Check sheet for the modelled part. Datum: model origin and axes. Units: mm. A direction names the side the tool comes from. Coordinates: 2 decimals unless noted, no trailing zeros. Loops run counter-clockwise (first coordinate to the right, second up) from the corner with the lowest first, then second, coordinate; pieces in that order, holes last. Notation, with made-up numbers: M -10.75,4.5 L 40.25,4.5 A28 cw 40.25,31.5 Z; hole C -10,22.25 d2. An arc over 180 degrees is marked long. Return JSON: item names as keys, results as strings.
from build123d import *

# Parameters (mm, degrees)
CROQUIS1_W              = 60
CROQUIS1_H              = 25
SALIENTE_EXTRUIR1_DEPTH = 25
CROQUIS2_R              = 22
CORTAR_EXTRUIR1_DEPTH   = 25
CROQUIS3_W              = 39.331186887
CROQUIS3_H              = 32.545982132
CORTAR_EXTRUIR6_DEPTH   = 5
CROQUIS6_W              = 71.754194534
CROQUIS6_H              = 47.315533904
CORTAR_EXTRUIR7_DEPTH   = 5
CROQUIS7_W              = 50
CROQUIS7_H              = 25
SALIENTE_EXTRUIR2_DEPTH = 2
CORTAR_EXTRUIR9_DEPTH   = 38
CORTAR_EXTRUIR11_DEPTH  = 31
CROQUIS11_W             = 1
CROQUIS11_H             = 2
SALIENTE_EXTRUIR3_DEPTH = 25
CORTAR_EXTRUIR12_DEPTH  = 25
SALIENTE_EXTRUIR4_DEPTH = 25
CROQUIS14_W             = 30
CROQUIS14_H             = 8
CORTAR_EXTRUIR15_DEPTH  = 22
REDONDEO4_R             = 5
REDONDEO5_R             = 5


with BuildPart() as part:
    # Croquis1 → Saliente-Extruir1 (new body)
    with BuildSketch(Plane(origin=(0, 0, 0), x_dir=(1, 0, 0), z_dir=(0, 1, 0))):
        Rectangle(CROQUIS1_W, CROQUIS1_H)
    extrude(amount=SALIENTE_EXTRUIR1_DEPTH)

    # Croquis2 → Cortar-Extruir1 (cut)
    with BuildSketch(Plane(origin=(0, 25, 0), x_dir=(1, 0, 0), z_dir=(0, 1, 0))):
        with Locations((0, 12.5)):
            Circle(CROQUIS2_R)
    extrude(amount=-CORTAR_EXTRUIR1_DEPTH, mode=Mode.SUBTRACT)

    # Croquis3 → Cortar-Extruir6 (cut)
    with BuildSketch(Plane(origin=(30, 0, 0), x_dir=(0, 0, -1), z_dir=(1, 0, 0))):
        with Locations((0.690020822, 11.469590882)):
            Rectangle(CROQUIS3_W, CROQUIS3_H)
    extrude(amount=-CORTAR_EXTRUIR6_DEPTH, mode=Mode.SUBTRACT)

    # Croquis6 → Cortar-Extruir7 (cut)
    with BuildSketch(Plane.ZY.offset(30)):
        with Locations((-5.334444443, 15.165040004)):
            Rectangle(CROQUIS6_W, CROQUIS6_H)
    extrude(amount=-CORTAR_EXTRUIR7_DEPTH, mode=Mode.SUBTRACT)

    # Croquis7 → Saliente-Extruir2 (add)
    with BuildSketch(Plane(origin=(0, 25, 0), x_dir=(1, 0, 0), z_dir=(0, 1, 0))):
        Rectangle(CROQUIS7_W, CROQUIS7_H)
    extrude(amount=SALIENTE_EXTRUIR2_DEPTH)

    # Croquis8 → Cortar-Extruir9 (cut)
    with BuildSketch(Plane(origin=(0, 0, -12.5), x_dir=(-1, 0, 0), z_dir=(0, 0, -1))):
        Polygon((-23.5, 0), (-23, 0), (-23, 3), (-24, 3), (-24, 0), align=None)
        Polygon((24, 0), (23.5, 0), (23, 0), (23, 3), (24, 3), align=None)
    extrude(amount=-CORTAR_EXTRUIR9_DEPTH, mode=Mode.SUBTRACT)

    # Croquis10 → Cortar-Extruir11 (cut)
    with BuildSketch(Plane(origin=(0, 0, -12.5), x_dir=(-1, 0, 0), z_dir=(0, 0, -1))):
        Polygon((23, 0), (24, 0), (24.465135072, 0), (24.465135072, 1), (22.465135072, 1), (22.465135072, 0), align=None)
        Polygon((-22.465135072, 0), (-22.465135072, 1), (-24.465135072, 1), (-24.465135072, 0), (-24, 0), (-23, 0), align=None)
    extrude(amount=-CORTAR_EXTRUIR11_DEPTH, mode=Mode.SUBTRACT)

    # Croquis11 → Saliente-Extruir3 (add)
    with BuildSketch(Plane(origin=(0, 0, -12.5), x_dir=(-1, 0, 0), z_dir=(0, 0, -1))):
        Polygon((22.465135072, 1), (22.465135072, 0), (24.465135072, 0), (24.465135072, 1), (24, 1), (23, 1), align=None)
        with Locations((23.5, 2)):
            Rectangle(CROQUIS11_W, CROQUIS11_H)
        Polygon((-23, 1), (-24, 1), (-24.465135072, 1), (-24.465135072, 0), (-22.465135072, 0), (-22.465135072, 1), align=None)
        with Locations((-23.5, 2)):
            Rectangle(CROQUIS11_W, CROQUIS11_H)
    extrude(amount=-SALIENTE_EXTRUIR3_DEPTH)

    # Croquis12 → Cortar-Extruir12 (cut)
    with BuildSketch(Plane(origin=(0, 0, -12.5), x_dir=(-1, 0, 0), z_dir=(0, 0, -1))):
        Polygon((-22.5, 0), (-24.5, 0), (-24.5, 1), (-24, 1), (-24, 3), (-23, 3), (-23, 1), (-22.5, 1), align=None)
        Polygon((24, 3), (23, 3), (23, 1), (22.5, 1), (22.5, 0), (24.5, 0), (24.5, 1), (24, 1), align=None)
    extrude(amount=-CORTAR_EXTRUIR12_DEPTH, mode=Mode.SUBTRACT)

    # Croquis13 → Saliente-Extruir4 (add)
    with BuildSketch(Plane(origin=(0, 0, -12.5), x_dir=(-1, 0, 0), z_dir=(0, 0, -1))):
        Polygon((-22, 0), (-22.5, 0), (-22.5, 1), (-23, 1), (-23, 3), (-24, 3), (-24, 1), (-24.5, 1), (-24.5, 0), (-25, 0), (-25, 27), (25, 27), (25, 0), (24.5, 0), (24.5, 1), (24, 1), (24, 3), (23, 3), (23, 1), (22.5, 1), (22.5, 0), (22, 0), (22, 25), (-22, 25), align=None)
    extrude(amount=SALIENTE_EXTRUIR4_DEPTH)

    # Croquis14 → Cortar-Extruir15 (cut)
    with BuildSketch(Plane.XY.offset(12.5)):
        with Locations((0, 10)):
            Rectangle(CROQUIS14_W, CROQUIS14_H)
    extrude(amount=-CORTAR_EXTRUIR15_DEPTH, mode=Mode.SUBTRACT)

    # Redondeo4
    redondeo4_edges = [part.edges().sort_by_distance(p)[0] for p in [
        (0, 25, 9.5),
        (-22, 25, -25),
        (22, 25, -25),
        (-25, 27, -12.5),
        (25, 27, -12.5),
    ]]
    fillet(redondeo4_edges, radius=REDONDEO4_R)

    # Redondeo5
    redondeo5_edges = [part.edges().sort_by_distance(p)[0] for p in [
        (-23.535533906, 25.535533906, 12.5),
        (23.535533906, 25.535533906, 12.5),
        (-25, 11, 12.5),
        (0, 27, 12.5),
        (25, 11, 12.5),
    ]]
    fillet(redondeo5_edges, radius=REDONDEO5_R)


solid = part.part
1) Section check B-B on y = 8. Record the cut outline in (x, z).
Answers:
{"outline": "M -25,-37.5 L -22,-37.5 L -22,-12.5 A22 cw -15,3.59 L -15,12.5 L -20,12.5 A5 ccw -25,7.5 Z; M 15,3.59 A22 cw 22,-12.5 L 22,-37.5 L 25,-37.5 L 25,7.5 A5 ccw 20,12.5 L 15,12.5 Z"}
2) Section check C-C on z = -29. Record the cut outline in (x, y), then the cut area to 3 significant figures.
Answers:
{"outline": "M -25,0 L -24.5,0 L -24.5,1 L -24,1 L -24,3 L -23,3 L -23,1 L -22.5,1 L -22.5,0 L -22,0 L -22,20 A5 cw -17,25 L 17,25 A5 cw 22,20 L 22,0 L 22.5,0 L 22.5,1 L 23,1 L 23,3 L 24,3 L 24,1 L 24.5,1 L 24.5,0 L 25,0 L 25,22 A5 ccw 20,27 L -20,27 A5 ccw -25,22 Z", "area": "242 mm²"}
3) Draft check along Y on faces 6 (the face through (-22, 10, -25)), 7 (the face through (15, 10, 8)), 8 (the face through (21, 23, -25)), 9 (the face through (-0.28, 25.5, 11.07)). Enter one of: +Y half, -Y half, draft (parallel to the pull), parting line (faces both ways), or undercut.
Answers:
{"face 6": "draft", "face 7": "undercut", "face 8": "-Y half", "face 9": "+Y half"}
4) Section check D-D on y = 5. Record the cut outline in (x, z), then the cut area to 3 significant figures.
Answers:
{"outline": "M -25,-37.5 L -22,-37.5 L -22,-12.5 A22 cw 22,-12.5 L 22,-37.5 L 25,-37.5 L 25,7.5 A5 ccw 20,12.5 L -20,12.5 A5 ccw -25,7.5 Z", "area": "629 mm²"}
5) Scan lines: line 1 along X through (y, z) = (17.5, -22); line 2 along Y through (x, z) = (14, 5); line 3 along Y through (x, z) = (-9, -16.5). Record each from-to range of solid material in increasing order. Write a range as [from, to].
Answers:
{"line 1": "[-25, -22], [22, 25]", "line 2": "[0, 6], [14, 27]", "line 3": "[25, 27]"}
6) Go/stop test with flat-tipped pins: pin 1 Ø7 at (x, z) = (4, 9) entering from +Y; pin 2 Ø1.5 at (x, y) = (7.5, 22.5) entering from -Z; pin 3 Ø4 at (x, z) = (-11, -30) entering from -Y; pin 4 Ø1.5 at (x, y) = (-12, 12.5) entering from -Z. Record where each tip stops, or that it passes through.
Answers:
{"pin 1": "y = 27", "pin 2": "z = 6.84", "pin 3": "y = 25", "pin 4": "through"}
7) Set-up check for faces 1 (the face through (0, 25, -16)), 2 (the face through (-15, 10, 8)), 3 (the face through (-23, 2, -13)), 4 (the face through (-23, 26, -15)), 5 (the face through (-2, 0, 10)): record each of +Z, -Z, +X, -X, +Y, -Y from which the full face is reachable in a straight line by a thin tool's end or side.
Answers:
{"face 1": "-Z, -Y", "face 2": "+Z, -Z", "face 3": "+Z, -Z, -Y", "face 4": "+Z, -Z, -X, +Y", "face 5": "+Z, -Z, +X, -X, -Y"}
8) Section check A-A on x = 0. Record the cut outline in (y, z).
Answers:
{"outline": "M 0,9.5 L 6,9.5 L 6,12.5 L 0,12.5 Z; M 14,9.5 L 20,9.5 A5 cw 25,4.5 L 25,-37.5 L 27,-37.5 L 27,7.5 A5 ccw 22,12.5 L 14,12.5 Z"}
